Geometry: see drawing. Coordinates: mm, zero at the bounding-box minimum. A direction names the side the tool comes from. Give positions to 0.01 mm unless a question says otherwise; leave off trailing zeros. Order: outer loops, then holes, each group sorted by start corner. A loop starts at its lowest first (then second) coordinate and runs counter-clockwise, first axis right, second up. Notation, with made-up numbers: (67, 21) -> (112, 21) arc R22 cw to (112, 60) -> close; hole circle Ø10 at (66.25, 31.25). An arc over 180 degrees is marked (long way). One line per item, written item: value. Start each with the question number.
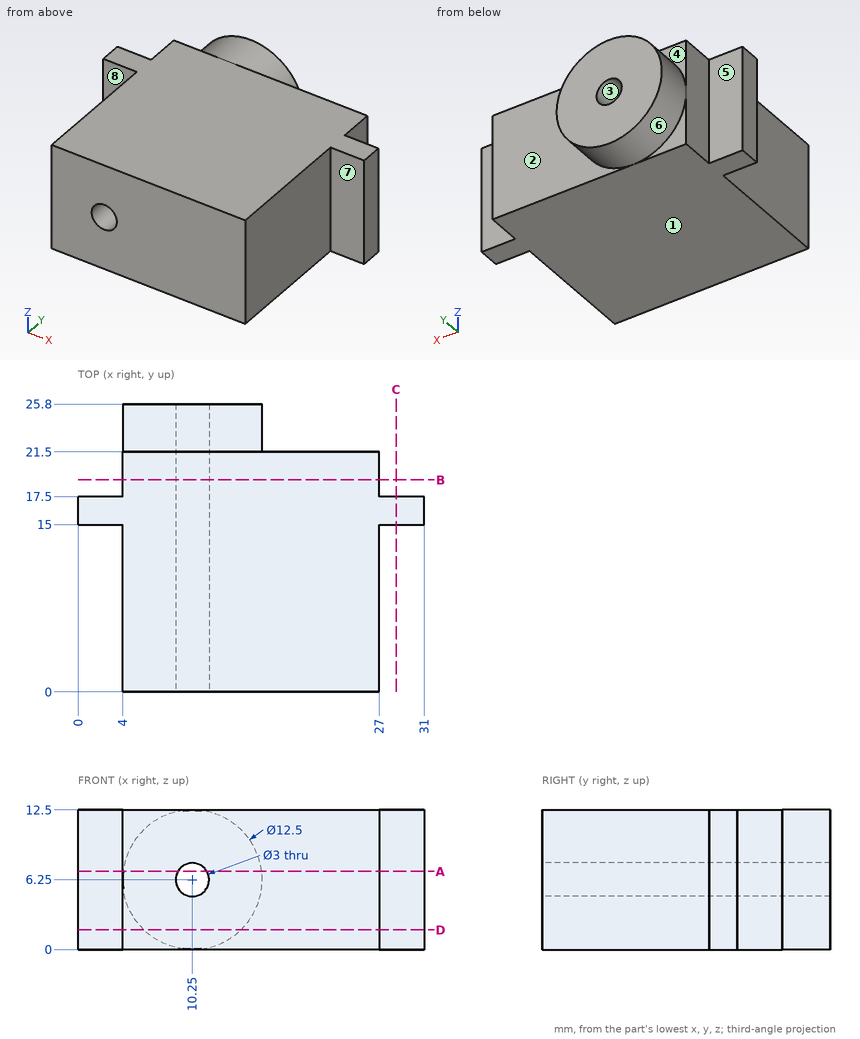
1. Access query for the marked faces 4, 5, 6, 7 and 8. Directions: +Z, -Z, +X, -X, +Y, -Y. A direction counts if a zero-diameter tool reaches every point of the face in a straight line with its end or side. Return the directions, or none.
2. Cut plane A-A, the plane z = 7. Return loops of the section in (x, y).
3. Material intervals for L1, parallel to Z at x = 10.25, y = 18.75; L2, parallel to X at y = 8, z = 6.25; L3, parallel to X at y = 17, z = 6.25, sorted ascending. Write a range as [from, to].
4. Cut plane B-B, the plane y = 19. Return loops of the section in (x, z), then the cut area to 3 significant figures.
5. Cut plane C-C, the plane x = 28.5. Return loops of the section in (y, z), then the cut area to 4 significant figures.
6. Draft query along Z for the marked faces 1, 2 and 3. Return one class per face: pulls with the +Z half, pulls with the -Z half, needs draft (parallel to the pull), parting line crosses it, or undercut.
7. Pin query (flat end, axial travel): P1, Ø1.2, axis at y = 19.5, z = 7.5, coming from the +X side; P2, Ø4.5, axis at x = 29, z = 6, coming from the +Y side; P3, Ø5, axis at y = 6, z = 10, coming from the -X side. Return the tip coordinate at first contact, or that it passes through.
8. Cut plane D-D, the plane z = 1.75. Return loops of the section in (x, y).
Answers follow:
1. face 4: +Z, -X, +Y
1. face 5: +Z, -Z, -X, +Y
1. face 6: +Y
1. face 7: +Z, -Z, +X, -Y
1. face 8: +Z, -Z, -X, -Y
2. outline: (0, 15) -> (4, 15) -> (4, 0) -> (8.95, 0) -> (8.95, 25.8) -> (4.05, 25.8) -> (4.05, 21.5) -> (4, 21.5) -> (4, 17.5) -> (0, 17.5) -> close; (11.55, 0) -> (27, 0) -> (27, 15) -> (31, 15) -> (31, 17.5) -> (27, 17.5) -> (27, 21.5) -> (16.45, 21.5) -> (16.45, 25.8) -> (11.55, 25.8) -> close
3. L1: z = [0, 4.75], [7.75, 12.5]
3. L2: x = [4, 8.75], [11.75, 27]
3. L3: x = [0, 8.75], [11.75, 31]
4. outline: (4, 0) -> (27, 0) -> (27, 12.5) -> (4, 12.5) -> close; hole circle Ø3 at (10.25, 6.25)
4. area: 280 mm²
5. outline: (15, 0) -> (17.5, 0) -> (17.5, 12.5) -> (15, 12.5) -> close
5. area: 31.25 mm²
6. face 1: pulls with the -Z half
6. face 2: needs draft
6. face 3: undercut
7. P1: stops at x = 27
7. P2: stops at y = 21.5
7. P3: stops at x = 4
8. outline: (0, 15) -> (4, 15) -> (4, 0) -> (27, 0) -> (27, 15) -> (31, 15) -> (31, 17.5) -> (27, 17.5) -> (27, 21.5) -> (14.59, 21.5) -> (14.59, 25.8) -> (5.91, 25.8) -> (5.91, 21.5) -> (4, 21.5) -> (4, 17.5) -> (0, 17.5) -> close
